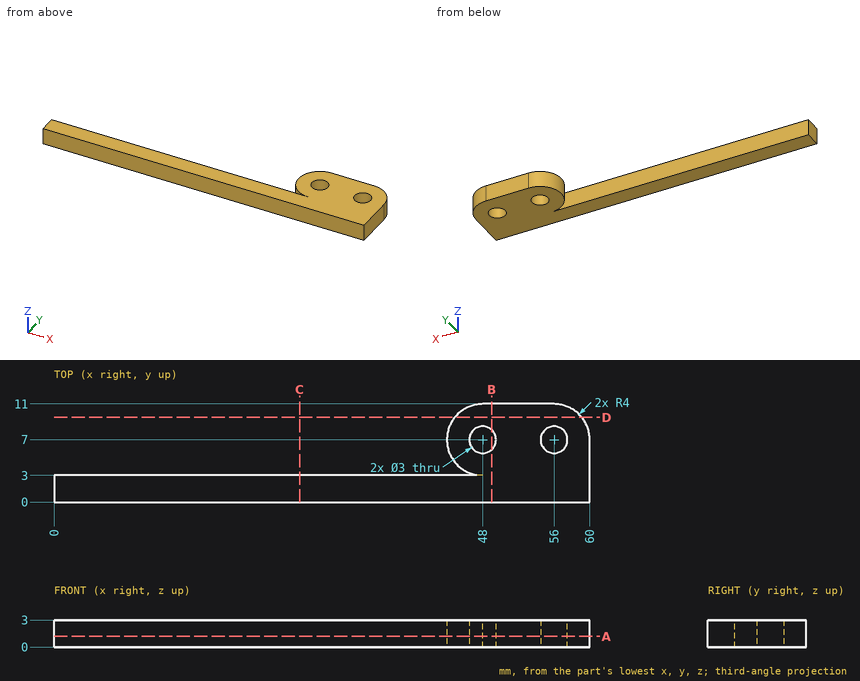
Drawing for the job (mm, zero at the part's lowest x, y, z). Give positions to 0.01 mm unless a question says otherwise; leave off trailing zeros. Loops run counter-clockwise (first coordinate to the right, second up) from the corner with the lowest first, then second, coordinate; pieces in that order, holes last. Notation, with made-up numbers: M -0.5,-35 L 16.5,-35 A23 cw 16.5,-6 Z; hole C 6.5,14 d3. An arc over 180 degrees is marked long. One line per question, with ' | ' between items. Start each with the question number.
1. Saw through at A-A on z = 1.2. Give the cut face in (x, y).
2. Saw through at B-B on x = 49. Give the cut face in (y, z), plus the area to 3 significant figures.
3. Saw through at D-D on y = 9.5. Give the cut face in (x, z).
4. Probe L1, parallel to Y at x = 56, z = 2.2; L2, parallel to X at y = 6.5, z = 0.95; L3, parallel to Y at x = 21.5, z = 0.6. List the from-to ranges inside material, lowest first. Write a range as from..to.
5. Saw through at C-C on x = 27.5. Give the cut face in (y, z), plus the area to 3 significant figures.
Result sheet:
1) outline: M 0,0 L 60,0 L 60,7 A4 ccw 56,11 L 48,11 A4 ccw 48,3 L 0,3 Z; hole C 48,7 d3; hole C 56,7 d3
2) outline: M 0,0 L 5.88,0 L 5.88,3 L 0,3 Z; M 8.12,0 L 11,0 L 11,3 L 8.12,3 Z | area: 26.3 mm^2
3) outline: M 44.88,0 L 59.12,0 L 59.12,3 L 44.88,3 Z
4) L1: y = 0..5.5, 8.5..11 | L2: x = 44.03..46.59, 49.41..54.59, 57.41..60 | L3: y = 0..3
5) outline: M 0,0 L 3,0 L 3,3 L 0,3 Z | area: 9.00 mm^2
